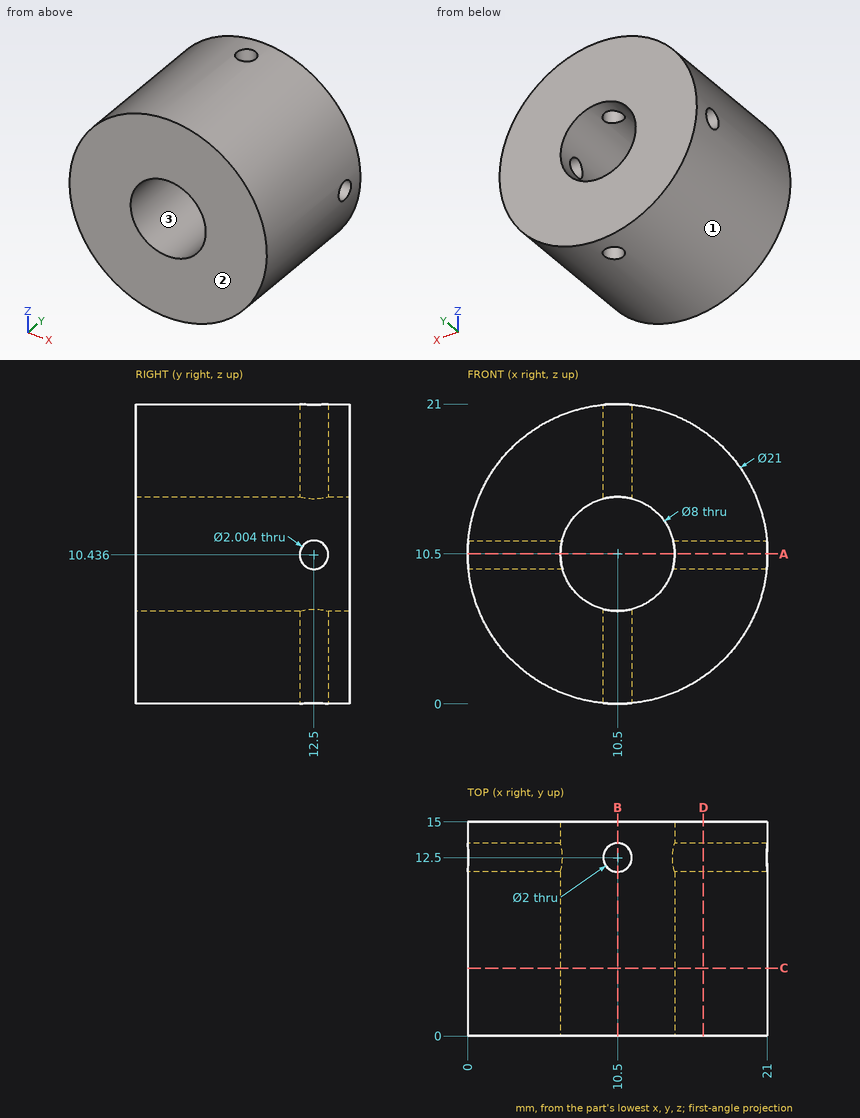
Answer from the drawing. Dimensions are ordinates in mm from the lowest x, y and z of the part. Coordinates: 2 decimals unless noted, no trailing zeros. Write each loop counter-clockwise with the first axis right and the second up, starting at its lowest first coordinate (ties: lowest second). Pieces come first, ordered by that corner, then holes. Notation, with made-up numbers: (19.25, 40) - (53.25, 40) arc R10 ccw to (53.25, 52) - close; hole circle Ø4 at (-36, 52). An arc over 180 degrees is marked (long way). Return JSON: item names as keys, results as strings. Group by question number.
Q1. The part is cut by section B-B on x = 10.5. Write down the section's boundary in (y, z).
Q2. The part is cut by section A-A on z = 10.5. Write down the section's boundary in (x, y), and give its area (3 significant figures).
Q3. The part is cut by section D-D on x = 16.5. Write down the section's boundary in (y, z) (1 decimal).
Q4. The part is cut by section C-C on y = 4.75. Write down the section's boundary in (x, z), and give its area (3 significant figures).
Q5. For a pull along X with two mould halves and no side action, classify the marked faces 1, 2 and 3 as +X half, -X half, draft (parallel to the pull), parting line (faces both ways), or undercut.
Q6. Flat-ended cylindrical pins translate along their axes: pin 1 Ø1 at (x, z) = (12, 11.5) entering from -Y; pin 2 Ø3 at (x, y) = (13.5, 3) entering from -Z; pin 3 Ø2 at (x, y) = (15.5, 12.5) entering from +Z; pin 4 Ø4 at (x, y) = (8, 5) entering from -Z. Find the tip coordinate at first contact, or state that the pin passes through.
Q7. Find the intervals of material crossed by line 1 along Z through (x, y) = (17, 11.75) (1 decimal); line 2 along X through (y, z) = (8.25, 13) (1 decimal); line 3 along Z through (x, y) = (7.5, 3.75) (1 decimal), in increasing order. Write a range as [from, to].
Evaluation:
{
 "1": {"outline": "(0, 0) - (11.5, 0) - (11.5, 6.5) - (0, 6.5) - close; (0, 14.5) - (11.5, 14.5) - (11.5, 21) - (0, 21) - close; (13.5, 0) - (15, 0) - (15, 6.5) - (13.5, 6.5) - close; (13.5, 14.5) - (15, 14.5) - (15, 21) - (13.5, 21) - close"},
 "2": {"outline": "(0, 0) - (6.5, 0) - (6.5, 11.5) - (0, 11.5) - close; (0, 13.5) - (6.5, 13.5) - (6.5, 15) - (0, 15) - close; (14.5, 0) - (21, 0) - (21, 11.5) - (14.5, 11.5) - close; (14.5, 13.5) - (21, 13.5) - (21, 15) - (14.5, 15) - close", "area": "169 mm2"},
 "3": {"outline": "(0, 1.9) - (15, 1.9) - (15, 19.1) - (0, 19.1) - close; hole circle Ø2 at (12.5, 10.4)"},
 "4": {"outline": "circle Ø21 at (10.5, 10.5); hole circle Ø8 at (10.5, 10.5)", "area": "296 mm2"},
 "5": {"face 1": "parting line", "face 2": "draft", "face 3": "undercut"},
 "6": {"pin 1": "passes through", "pin 2": "stops at z = 0.11", "pin 3": "stops at z = 20.21", "pin 4": "stops at z = 0.01"},
 "7": {"line 1": "z = [2.3, 9.8], [11.1, 18.7]", "line 2": "x = [0.3, 7.4], [13.6, 20.7]", "line 3": "z = [0.4, 7.9], [13.1, 20.6]"}
}
